Here's how the part is built. I have some questions about the finished solid (model axes, mm). Coordinates: 2 decimals unless noted, no trailing zeros. Write each loop counter-clockwise with the first axis right and the second up, starting at its lowest first coordinate (ties: lowest second). Pieces come first, ordered by that corner, then holes. Notation, with made-up numbers: (-31.75, 39.25) -> (22.25, 39.25) arc R20 ccw to (22.25, 44.25) -> close; hole circle Ø6 at (45, -36.75). An arc over 180 degrees is marked (long way). Use a Markdown table: item, result. Add a question column.
Item 1: Imagine slicing it at B-B, the plane y = 0.9. Count the separate pieces of the cut face and the enclosed holes in it, and give its area (3 significant figures).
Item 2: Imagine slicing it at D-D, the plane z = 40. Write out the boundary of the cut face in (x, y), and give its area (3 significant figures).
Item 3: Imagine slicing it at C-C, the plane x = -8.5. Write out the boundary of the cut face in (y, z), and give its area (3 significant figures).
Item 4: Will these pins go through, and if not, where does the flat tip stop? pin 1 Ø1.2 at (y, z) = (3, -36.5) entering from -X; pin 2 Ø1.2 at (y, z) = (2, -38) entering from +X; pin 3 Ø1.2 at (x, y) = (111, 2) entering from -Z.
Item 5: If I drill on line 1 along X through (y, z) = (2.4, 5); line 2 along Z through (x, y) = (-18.5, 3.25); line 3 along X through (y, z) = (2.7, -43), over which ranges is the centre line in solid material (lowest first)? Write a range as from..to.
Item 6: Imagine slicing it at A-A, the plane z = 0. Write out the boundary of the cut face in (x, y).
```python
from build123d import *

# Parameters (mm, degrees)
EXTRUDE_1_DEPTH     = 4
FILLET_1_R          = 5
FILLET_2_R          = 20
FILLET_3_R          = 5
SKETCH_2_R          = 8
CUT_EXTRUDE_1_DEPTH = 10
CUT_EXTRUDE_2_DEPTH = 10


with BuildPart() as part:
    # 草图1 → 凸台-拉伸1 (new body)
    with BuildSketch(Plane(origin=(0, 0, 0), x_dir=(1, 0, 0), z_dir=(0, 1, 0))):
        Polygon((90, 54), (90, 29), (160, 29), (160, -50), (-160, -50), (-160, 29), (-90, 29), (-90, 54), align=None)
    extrude(amount=EXTRUDE_1_DEPTH)

    # 圆角1
    fillet_1_edges = [part.edges().sort_by_distance(p)[0] for p in [
        (-90, 2, -29),
        (-90, 2, -54),
        (90, 2, -54),
        (90, 2, -29),
    ]]
    fillet(fillet_1_edges, radius=FILLET_1_R)

    # 圆角2
    fillet_2_edges = [part.edges().sort_by_distance(p)[0] for p in [
        (160, 2, 50),
        (-160, 2, 50),
    ]]
    fillet(fillet_2_edges, radius=FILLET_2_R)

    # 圆角3
    fillet_3_edges = [part.edges().sort_by_distance(p)[0] for p in [
        (-160, 2, -29),
        (160, 2, -29),
    ]]
    fillet(fillet_3_edges, radius=FILLET_3_R)

    # 草图2 → 切除-拉伸1 (cut)
    with BuildSketch(Plane.XZ):
        with Locations(Location((12.499997526, 0.007864027, 0), (0, 0, 270))):
            Circle(SKETCH_2_R)
        with Locations(Location((-12.499997526, -0.007864027, 0), (0, 0, 270))):
            Circle(SKETCH_2_R)
    extrude(amount=-CUT_EXTRUDE_1_DEPTH, mode=Mode.SUBTRACT)

    # 草图4 → 切除-拉伸2 (cut)
    with BuildSketch(Plane(origin=(0, 4, 0), x_dir=(1, 0, 0), z_dir=(0, 1, 0))):
        with BuildLine():
            Line((-2.1, 35), (-2.1, 40))
            ThreePointArc((-2.1, 40), (0, 42.1), (2.1, 40))
            Line((2.1, 40), (2.1, 35))
            ThreePointArc((2.1, 35), (0, 32.9), (-2.1, 35))
        make_face()
        with BuildLine():
            Line((62.1, 35), (62.1, 40))
            ThreePointArc((62.1, 40), (60, 42.1), (57.9, 40))
            Line((57.9, 40), (57.9, 35))
            ThreePointArc((57.9, 35), (60, 32.9), (62.1, 35))
        make_face()
        with BuildLine():
            Line((-57.9, 35), (-57.9, 40))
            ThreePointArc((-57.9, 40), (-60, 42.1), (-62.1, 40))
            Line((-62.1, 40), (-62.1, 35))
            ThreePointArc((-62.1, 35), (-60, 32.9), (-57.9, 35))
        make_face()
    extrude(amount=-CUT_EXTRUDE_2_DEPTH, mode=Mode.SUBTRACT)


solid = part.part
```
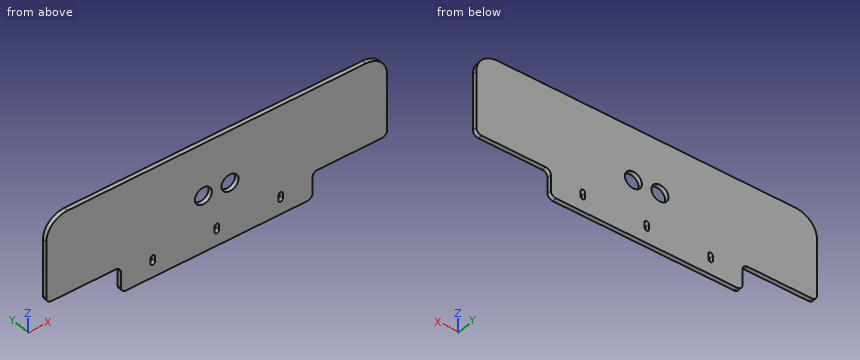
Ans:
| question | item | result |
|---|---|---|
| 1 | separate pieces | 1 |
| 1 | enclosed holes | 5 |
| 1 | area | 29,100 mm^2 |
| 2 | outline | (-157.32, 0) -> (157.32, 0) -> (157.32, 4) -> (-157.32, 4) -> close |
| 2 | area | 1,260 mm^2 |
| 3 | outline | (0, -54) -> (4, -54) -> (4, -6.94) -> (0, -6.94) -> close; (0, 6.92) -> (4, 6.92) -> (4, 50) -> (0, 50) -> close |
| 3 | area | 361 mm^2 |
| 4 | pin 1 | stops at x = -90 |
| 4 | pin 2 | stops at x = 90 |
| 4 | pin 3 | stops at z = -29 |
| 5 | line 1 | x = -160..-18.74, -6.26..6.25, 18.75..160 |
| 5 | line 2 | z = -54..-5.3, 5.28..50 |
| 5 | line 3 | x = -90..90 |
| 6 | outline | (-160, 0) -> (-20.5, 0) -> (-20.5, 4) -> (-160, 4) -> close; (-4.5, 0) -> (4.5, 0) -> (4.5, 4) -> (-4.5, 4) -> close; (20.5, 0) -> (160, 0) -> (160, 4) -> (20.5, 4) -> close |
